Part model, mm, in its own coordinate system. A direction names the side the tool comes from. Give positions to 0.01 mm unless a question says otherwise; leave off trailing zeros. Order: outer loops, then holes, each group sorted by start corner. A loop starts at its lowest first (then second) coordinate and runs counter-clockwise, first axis right, second up. Notation, with made-up numbers: (69, 51) -> (99, 51) arc R18 cw to (99, 80) -> close; hole circle Ø8 at (40.25, -12). An arc over 180 degrees is marked (long way). Write item = value, one per line. Start each with the question number.
(1) Flat gauge pins, fed straight in: pin 1 (3 mm diameter, centred on x = 13.5, z = -13, fed in from -Y); pin 2 (12 mm diameter, centred on x = -51.5, y = 46, fed in from +Z); pin 3 (18 mm diameter, centred on x = 0, y = 0, fed in from -Z); pin 4 (1 mm diameter, centred on x = -19.5, z = -13.5, fed in from -Y). Where does each tip first touch, or does it go through?
(2) Two-plate mould, pull along Y, no slides. Class faces 1 (the cylindrical face through (-64.49, 59.14, -7.89)), 2 (the flat face through (18, 1, -16)), 3 (the flat face through (22, 0, -5)), 4 (the flat face through (0, 22, -5)): pulls with the +Y half, pulls with the -Y half, needs draft (parallel to the pull), parting line crosses it, or undercut.
(3) Probe line 1 along Y through (x, z) = (0, -2.25); line 2 along X through (y, z) = (-18.5, -7); line 3 along Y through (x, z) = (0, -11.75). List the from-to ranges inside material, lowest first. Write a range as from..to.
(4) Saw through at B-B, the plane x = 0. List the corners of the cut face in (y, z), then the cut area to 3 significant figures.
(5) Saw through at A-A, the plane z = -6.75. List the corners of the cut face in (x, y), then the cut area to 3 significant figures.
(6) Saw through at D-D, the plane x = 31. List the corners of the cut face in (y, z), then the cut area to 3 significant figures.
(7) Which spindle directions (+Z, -Z, +X, -X, +Y, -Y) get a long thin tool onto all of the face, cutting with end or side? Do faces 5 (the flat face through (-59, 59, 0)), 6 (the flat face through (-22, 0, -5)). Say none if no direction does.
from build123d import *

# Parameters (mm, degrees)
F0_R     = 87.5
F0_R_2   = 82.5
F0_R_3   = 15
F1_DEPTH = 16
F2_DEPTH = 10
F3_W     = 44
F3_H     = 44
F3_R     = 15
F4_DEPTH = 10
F5_SIZE  = 2


with BuildPart() as f1:
    # F0 (on Top) → F1 (new body)
    with BuildSketch(Plane.XY):
        Circle(F0_R)
        Circle(F0_R_2, mode=Mode.SUBTRACT)
        Circle(F0_R_2)
        Circle(F0_R_3, mode=Mode.SUBTRACT)
    extrude(amount=-F1_DEPTH)

    # F0 (on Top) → F2 (cut)
    with BuildSketch(Plane.XY):
        Circle(F0_R_2)
        Circle(F0_R_3, mode=Mode.SUBTRACT)
    extrude(amount=-F2_DEPTH, mode=Mode.SUBTRACT)

    # F3 (on face) → F4 (join)
    with BuildSketch(Plane.XY.offset(-10)):
        Rectangle(F3_W, F3_H)
        Circle(F3_R, mode=Mode.SUBTRACT)
    extrude(amount=F4_DEPTH)

    # F5
    f5_edges = [f1.edges().sort_by_distance(p)[0] for p in [
        (22, -22, -5),
        (-22, -22, -5),
        (22, 22, -5),
        (-22, 22, -5),
    ]]
    chamfer(f5_edges, length=F5_SIZE)


solid = f1.part
Results list:
q1.pin_1 = -86.67
q1.pin_2 = -10
q1.pin_3 = through
q1.pin_4 = -85.41
q2.face_1 = parting line crosses it
q2.face_2 = needs draft
q2.face_3 = undercut
q2.face_4 = undercut
q3.line_1 = -87.5..-82.5, -22..-15, 15..22, 82.5..87.5
q3.line_2 = -85.52..-80.4, -22..22, 80.4..85.52
q3.line_3 = -87.5..-15, 15..87.5
q4.outline = (-87.5, -16) -> (-15, -16) -> (-15, 0) -> (-22, 0) -> (-22, -10) -> (-82.5, -10) -> (-82.5, 0) -> (-87.5, 0) -> close; (15, -16) -> (87.5, -16) -> (87.5, 0) -> (82.5, 0) -> (82.5, -10) -> (22, -10) -> (22, 0) -> (15, 0) -> close
q4.area = 1,110 mm^2
q5.outline = circle Ø175 at (0, 0); (-22, -20) -> (-20, -22) -> (20, -22) -> (22, -20) -> (22, 20) -> (20, 22) -> (-20, 22) -> (-22, 20) -> close; hole circle Ø165 at (0, 0); hole circle Ø30 at (0, 0)
q5.area = 3,890 mm^2
q6.outline = (-81.82, -16) -> (81.82, -16) -> (81.82, 0) -> (76.45, 0) -> (76.45, -10) -> (-76.45, -10) -> (-76.45, 0) -> (-81.82, 0) -> close
q6.area = 1,090 mm^2
q7.face_5 = +Z, +X, -X, +Y, -Y
q7.face_6 = +Z
